Model file for the job. Use its own axes, mm. Face numbers are marked on the shaded views. A direction names the side the tool comes from. Round coordinates to 2 decimals unless told otherwise and drop trailing zeros. Order: outer loops, then holes, each group sorted by start corner. A loop starts at its lowest first (then second) coordinate and runs counter-clockwise, first axis right, second up. Notation, with made-up numbers: (3.25, -8) -> (33.25, -8) arc R28 cw to (33.25, 19) -> close; hole circle Ø7 at (-13.75, -30). An arc over 180 degrees is marked (long way). Put each result on its own line as item: value. Start each with the question number.
Q1. Probe L1, parallel to Z at x = -5.25, y = 92.45; L2, parallel to X at y = 93.3, z = -12; L3, parallel to X at y = 90.45, z = -27. List the from-to ranges inside material, lowest first.
Q2. Cut at A-A, the plane z = -13. List the corners of the cut face in (x, y).
Q3. Cut at C-C, the plane x = -6.75. List the corners of the cut face in (y, z).
Q4. 3-axis set-ups, long thin cutter, end or side, ignore diameter. For the marked faces 1, 2, 3 and 4: which of +Z, -Z, +X, -X, +Y, -Y reach the whole face in a straight line?
Q5. Flat gauge pins, fed straight in: P1, Ø2, axis at x = 9, y = 93.5, coming from the +Z side; P2, Ø4, axis at x = -5.5, z = -2.5, coming from the -Y side; P3, Ø2, axis at x = 7, y = 90.5, coming from the -Z side. Where does each tip first touch, or does it go through?
Q6. Cut at B-B, the plane x = 0. List the corners of the cut face in (y, z) (3 decimals), and give its area (3 significant figures).
Q7. Pull direction Z, two halves, no side cores. Call the marked faces 5, 6 and 7: released by +Z, released by -Z, zero draft, split by the parting line, or undercut.
Q8. Cut at D-D, the plane y = 93.4. State how many separate pieces and enclosed holes the cut face has, and give its area (3 significant figures).
from build123d import *
from build123d.topology import SkipClean

# Parameters (mm, degrees)
BATTERY_HOLDER_OUTLINE_DEPTH        = 2
LIP_START                           = 2
LIP_DEPTH                           = 2
SKETCH4_R                           = 1
SCREWHOLE_DEPTH                     = 10
SKETCH5_W                           = 18
SKETCH5_H                           = 15
ACTUAL_BATTERY_CAP_THINGY_DEPTH     = 1.5
FILLETS_START                       = 91.999999219
FILLETS_FOR_THE_THING_ABOVE_DEPTH   = 2.000000781
FILLETS_START_2                     = -12
FILLETS_FOR_THE_THING_ABOVE_2_DEPTH = 23
FILLETS_AT_EDGE_R                   = 2


with BuildPart() as part:
    # Sketch2 → Battery holder outline (new body)
    with BuildSketch(Plane(origin=(0, 92, 0), x_dir=(1, 0, 0), z_dir=(0, 1, 0))):
        with BuildLine():
            Line((-9.5, -18), (-4.5, -18))
            ThreePointArc((-4.5, -18), (-3.085786438, -18.585786438), (-2.5, -20))
            Line((-2.5, -20), (-2.5, -29.579540649))
            ThreePointArc((-2.5, -29.579540649), (0, -29.685), (2.5, -29.579540649))
            Line((2.5, -29.579540649), (2.5, -20))
            ThreePointArc((2.5, -20), (3.085786438, -18.585786438), (4.5, -18))
            Line((4.5, -18), (9.5, -18))
            ThreePointArc((9.5, -18), (11.267766953, -17.267766953), (12, -15.5))
            Line((12, -15.5), (12, 15.5))
            ThreePointArc((12, 15.5), (11.267766953, 17.267766953), (9.5, 18))
            Line((9.5, 18), (4.5, 18))
            ThreePointArc((4.5, 18), (3.085786438, 18.585786438), (2.5, 20))
            Line((2.5, 20), (2.5, 29.579540649))
            ThreePointArc((2.5, 29.579540649), (0, 29.685), (-2.5, 29.579540649))
            Line((-2.5, 29.579540649), (-2.5, 20))
            ThreePointArc((-2.5, 20), (-3.085786438, 18.585786438), (-4.5, 18))
            Line((-4.5, 18), (-9.5, 18))
            ThreePointArc((-9.5, 18), (-11.267766953, 17.267766953), (-12, 15.5))
            Line((-12, 15.5), (-12, -15.5))
            ThreePointArc((-12, -15.5), (-11.267766953, -17.267766953), (-9.5, -18))
        make_face()
        with BuildLine():
            Line((8, 15), (-8, 15))
            ThreePointArc((-8, 15), (-8.707106781, 14.707106781), (-9, 14))
            Line((-9, 14), (-9, -14))
            ThreePointArc((-9, -14), (-8.707106781, -14.707106781), (-8, -15))
            Line((-8, -15), (8, -15))
            ThreePointArc((8, -15), (8.707106781, -14.707106781), (9, -14))
            Line((9, -14), (9, 14))
            ThreePointArc((9, 14), (8.707106781, 14.707106781), (8, 15))
        make_face(mode=Mode.SUBTRACT)
    extrude(amount=BATTERY_HOLDER_OUTLINE_DEPTH)

    # Sketch3 → Lip (add)
    with SkipClean():  # the faces are left unmerged after this step: merging them gives an invalid solid
        with BuildSketch(Plane.XZ.offset(-92).offset(LIP_START)):
            with BuildLine():
                Line((2.5, 20), (2.5, 29.579540649))
                ThreePointArc((2.5, 29.579540649), (1.875417387, 29.625698888), (1.25, 29.658670317))
                Line((1.25, 29.658670317), (1.25, 28.407511771))
                Line((1.25, 28.407511771), (1.25, 20))
                ThreePointArc((1.25, 20), (2.201902961, 17.701902961), (4.5, 16.75))
                Line((4.5, 16.75), (9.5, 16.75))
                ThreePointArc((9.5, 16.75), (10.383883476, 16.383883476), (10.75, 15.5))
                Line((10.75, 15.5), (10.75, -15.5))
                ThreePointArc((10.75, -15.5), (10.383883476, -16.383883476), (9.5, -16.75))
                Line((9.5, -16.75), (4.5, -16.75))
                ThreePointArc((4.5, -16.75), (2.201902961, -17.701902961), (1.25, -20))
                Line((1.25, -20), (1.25, -28.407511771))
                Line((1.25, -28.407511771), (1.25, -29.658670317))
                ThreePointArc((1.25, -29.658670317), (1.875417387, -29.625698888), (2.5, -29.579540649))
                Line((2.5, -29.579540649), (2.5, -20))
                ThreePointArc((2.5, -20), (3.085786438, -18.585786438), (4.5, -18))
                Line((4.5, -18), (9.5, -18))
                ThreePointArc((9.5, -18), (11.267766953, -17.267766953), (12, -15.5))
                Line((12, -15.5), (12, 15.5))
                ThreePointArc((12, 15.5), (11.267766953, 17.267766953), (9.5, 18))
                Line((9.5, 18), (4.5, 18))
                ThreePointArc((4.5, 18), (3.085786438, 18.585786438), (2.5, 20))
            make_face()
            with BuildLine():
                Line((-2.5, -20), (-2.5, -29.579540649))
                ThreePointArc((-2.5, -29.579540649), (-1.875417387, -29.625698888), (-1.25, -29.658670317))
                Line((-1.25, -29.658670317), (-1.25, -28.407511771))
                Line((-1.25, -28.407511771), (-1.25, -20))
                ThreePointArc((-1.25, -20), (-2.201902961, -17.701902961), (-4.5, -16.75))
                Line((-4.5, -16.75), (-9.5, -16.75))
                ThreePointArc((-9.5, -16.75), (-10.383883476, -16.383883476), (-10.75, -15.5))
                Line((-10.75, -15.5), (-10.75, 15.5))
                ThreePointArc((-10.75, 15.5), (-10.383883476, 16.383883476), (-9.5, 16.75))
                Line((-9.5, 16.75), (-4.5, 16.75))
                ThreePointArc((-4.5, 16.75), (-2.201902961, 17.701902961), (-1.25, 20))
                Line((-1.25, 20), (-1.25, 28.407511771))
                Line((-1.25, 28.407511771), (-1.25, 29.658670317))
                ThreePointArc((-1.25, 29.658670317), (-1.875417387, 29.625698888), (-2.5, 29.579540649))
                Line((-2.5, 29.579540649), (-2.5, 20))
                ThreePointArc((-2.5, 20), (-3.085786438, 18.585786438), (-4.5, 18))
                Line((-4.5, 18), (-9.5, 18))
                ThreePointArc((-9.5, 18), (-11.267766953, 17.267766953), (-12, 15.5))
                Line((-12, 15.5), (-12, -15.5))
                ThreePointArc((-12, -15.5), (-11.267766953, -17.267766953), (-9.5, -18))
                Line((-9.5, -18), (-4.5, -18))
                ThreePointArc((-4.5, -18), (-3.085786438, -18.585786438), (-2.5, -20))
            make_face()
        extrude(amount=-LIP_DEPTH)

    # Sketch4 → Screwhole (cut)
    with SkipClean():  # the faces are left unmerged after this step: merging them gives an invalid solid
        with BuildSketch(Plane(origin=(0, 94, 0), x_dir=(1, 0, 0), z_dir=(0, 1, 0))):
            with Locations(Location((0, 17, 0), (0, 0, 270))):
                Circle(SKETCH4_R)
            with Locations(Location((0, -17, 0), (0, 0, 270))):
                Circle(SKETCH4_R)
        extrude(amount=-SCREWHOLE_DEPTH, mode=Mode.SUBTRACT)

    # Sketch5 → Actual battery cap thingy (add)
    with SkipClean():  # the faces are left unmerged after this step: merging them gives an invalid solid
        with BuildSketch(Plane(origin=(0, 94, 0), x_dir=(1, 0, 0), z_dir=(0, 1, 0))):
            Rectangle(SKETCH5_W, SKETCH5_H)
        extrude(amount=-ACTUAL_BATTERY_CAP_THINGY_DEPTH)

    # Fillets for the thing above: read off the stored shape, not the designer's step
    # Fillets for the thing above outline → Fillets for the thing above (add)
    with SkipClean():  # the faces are left unmerged after this step: merging them gives an invalid solid
        with BuildSketch(Plane(origin=(0, 0, 0), x_dir=(1, 0, 0), z_dir=(0, 1, 0)).offset(FILLETS_START)):
            with BuildLine():
                ThreePointArc((9, 10.5), (8.121320344, 8.378679656), (6, 7.5))
                Line((6, 7.5), (-6, 7.5))
                ThreePointArc((-6, 7.5), (-8.121320344, 8.378679656), (-9, 10.5))
                Line((-9, 10.5), (-9, -10.5))
                ThreePointArc((-9, -10.5), (-8.121320344, -8.378679656), (-6, -7.5))
                Line((-6, -7.5), (6, -7.5))
                ThreePointArc((6, -7.5), (8.121320344, -8.378679656), (9, -10.5))
                Line((9, -10.5), (9, 10.5))
            make_face()
        extrude(amount=FILLETS_FOR_THE_THING_ABOVE_DEPTH)

    # Fillets for the thing above 2 outline → Fillets for the thing above 2 (cut)
    with SkipClean():  # the faces are left unmerged after this step: merging them gives an invalid solid
        with BuildSketch(Plane.XY.offset(FILLETS_START_2)):
            with BuildLine():
                ThreePointArc((9.000010237, 91.99999321), (8.207718889, 92.37227955), (7.341687605, 92.5))
                Line((7.341687605, 92.5), (-7.341687605, 92.5))
                ThreePointArc((-7.341687605, 92.5), (-8.207718889, 92.37227955), (-9.000010237, 91.99999321))
                Line((-9.000010237, 91.99999321), (9.000010237, 91.99999321))
            make_face()
        extrude(amount=FILLETS_FOR_THE_THING_ABOVE_2_DEPTH, mode=Mode.SUBTRACT)

    # Fillets at edge
    # the kernel refuses this fillet: 2 mm, written as the material it takes off along each edge
    with BuildSketch(Plane(origin=(-1.25, 85.167051774, -29.658670317), x_dir=(-0.9980023206455083, 0, 0.06317727428577244), z_dir=(0, 1, 0)), Plane(origin=(1.25, 85.167051774, 29.658670317), x_dir=(0.9980023206455083, 0, -0.06317727428577508), z_dir=(0, 1, 0))) as fillets_at_edge_piece_1:
        with BuildLine():
            CenterArc((2.11813764, 1.802962869), FILLETS_AT_EDGE_R, 176.377796501, 67.975687163)
            Line((0.122132998, 1.929317418), (0, 0))
            ThreePointArc((0, 0), (0.626251049, -0.006606603), (1.252502098, 0))
        make_face()
    extrude(amount=6.832948226, mode=Mode.SUBTRACT)
    with BuildSketch(Plane(origin=(1.25, 85.167051774, -29.658670317), x_dir=(0.998002320645508, 0, 0.06317727428577799), z_dir=(0, 1, 0)), Plane(origin=(-1.25, 85.167051774, 29.658670317), x_dir=(-0.998002320645508, 0, -0.06317727428577828), z_dir=(0, 1, 0))) as fillets_at_edge_piece_2:
        with BuildLine():
            CenterArc((2.11813764, -1.802962869), FILLETS_AT_EDGE_R, 115.646516337, 67.975687163)
            Line((0.122132998, -1.929317418), (0, 0))
            ThreePointArc((0, 0), (0.626251049, 0.006606603), (1.252502098, 0))
        make_face()
    extrude(amount=6.832948226, mode=Mode.SUBTRACT)


solid = part.part
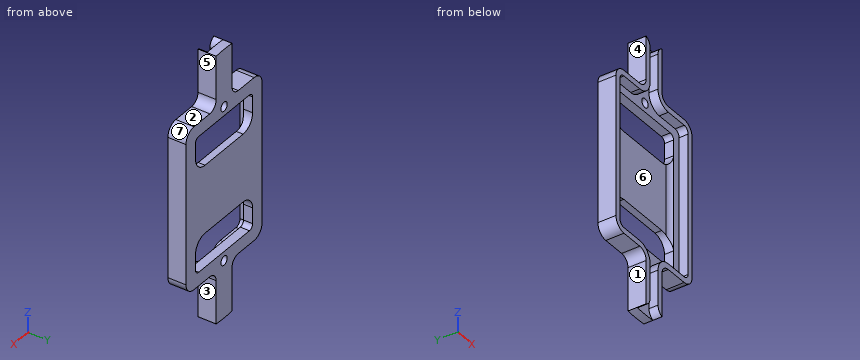
Ans:
1. L1: z = -18 to -15, 15 to 18
1. L2: x = -12 to -9, 9 to 12
1. L3: x = -2.5 to -1.25, 1.25 to 2.5
2. outline: (-12, 90) -> (-10.75, 90) -> (-10.75, 92) -> (-9, 92) -> (-9, 94) -> (-12, 94) -> close; (9, 92) -> (10.75, 92) -> (10.75, 90) -> (12, 90) -> (12, 94) -> (9, 94) -> close
3. outline: (90, -18) -> (94, -18) -> (94, -15) -> (92, -15) -> (92, -16.75) -> (90, -16.75) -> close; (90, 16.75) -> (92, 16.75) -> (92, 15) -> (94, 15) -> (94, 18) -> (90, 18) -> close; (92.5, -7.6) -> (94, -7.6) -> (94, 7.6) -> (92.5, 7.6) -> close
4. face 1: -Z, -X, +Y, -Y
4. face 2: +Z, +X, +Y, -Y
4. face 3: -Z, +X, +Y, -Y
4. face 4: +Z, -X, +Y, -Y
5. P1: stops at z = 18
5. P2: stops at y = 92.5
5. P3: stops at z = -18
6. outline: (92, -29.685) -> (94, -29.685) -> (94, -18) -> (92, -18) -> close; (92, -16) -> (94, -16) -> (94, -15) -> (92, -15) -> close; (92, 15) -> (94, 15) -> (94, 16) -> (92, 16) -> close; (92, 18) -> (94, 18) -> (94, 29.685) -> (92, 29.685) -> close; (92.5, -7.5) -> (94, -7.5) -> (94, 7.5) -> (92.5, 7.5) -> close
6. area: 73.2 mm^2
7. face 5: zero draft
7. face 6: undercut
7. face 7: released by +Z
8. separate pieces: 1
8. enclosed holes: 4
8. area: 711 mm^2
